Verification items for the finished model (mm, model axes). A direction names the side the tool comes from. Round coordinates to 2 decimals unless told otherwise and drop trailing zeros. Order: outer loops, then holes, each group sorted by start corner. A loop starts at its lowest first (then second) coordinate and runs counter-clockwise, first axis right, second up. Notation, with made-up numbers: M -19,26.5 L -5,26.5 A20 ccw -5,60.5 Z; hole C -21.5,3.5 d7. An arc over 180 degrees is marked long. Answer as a JSON object with one key per item and string values. Group by question number.
```python
from build123d import *

# Parameters (mm, degrees)
SKETCH_1_W          = 110
SKETCH_1_H          = 20
SKETCH_1_R          = 1.7
EXTRUDE_1_DEPTH     = 4.5
SKETCH_2_W          = 20
SKETCH_2_H          = 8
EXTRUDE_2_DEPTH     = 45
SKETCH_4_W          = 10
SKETCH_4_H          = 10
EXTRUDE_3_DEPTH     = 4.5
SKETCH_5_R          = 1.9
SKETCH_5_R_2        = 1.7
CUT_EXTRUDE_1_DEPTH = 75.885745444
CUT_EXTRUDE_2_DEPTH = 1.3
CUT_EXTRUDE_3_DEPTH = 2.6
SKETCH_7_R          = 1.7
CUT_EXTRUDE_5_DEPTH = 78.673192742
CUT_EXTRUDE_6_DEPTH = 1.3
SKETCH_9_W          = 80
SKETCH_9_H          = 3
EXTRUDE_4_DEPTH     = 50
SKETCH_11_W         = 17.2
SKETCH_11_H         = 50
SKETCH_11_W_2       = 9.3
SKETCH_11_R         = 2.5
SKETCH_11_R_2       = 1.7
CUT_EXTRUDE_7_DEPTH = 90.304255218
RIB_4_REACH         = 124.026
SKETCH_12_WALL_W    = 285.10321006
SKETCH_12_WALL_H    = 2
FILLET_1_R          = 2
FILLET_2_R          = 1.5
FILLET_3_R          = 2


with BuildPart() as part:
    # 草图1 → 凸台-拉伸1 (new body)
    with BuildSketch(Plane.XY):
        with Locations((0, 10)):
            Rectangle(SKETCH_1_W, SKETCH_1_H)
        with Locations((-45, 14)):
            Circle(SKETCH_1_R, mode=Mode.SUBTRACT)
        with Locations((-30, 14)):
            Circle(SKETCH_1_R, mode=Mode.SUBTRACT)
        with Locations((-15, 14)):
            Circle(SKETCH_1_R, mode=Mode.SUBTRACT)
        with Locations((15, 14)):
            Circle(SKETCH_1_R, mode=Mode.SUBTRACT)
        with Locations((30, 14)):
            Circle(SKETCH_1_R, mode=Mode.SUBTRACT)
        with Locations((45, 14)):
            Circle(SKETCH_1_R, mode=Mode.SUBTRACT)
    extrude(amount=EXTRUDE_1_DEPTH)

    # 草图2 → 凸台-拉伸2 (add)
    with BuildSketch(Plane.XY.offset(4.5)):
        with Locations((-45, 4)):
            Rectangle(SKETCH_2_W, SKETCH_2_H)
        with Locations((45, 4)):
            Rectangle(SKETCH_2_W, SKETCH_2_H)
    extrude(amount=EXTRUDE_2_DEPTH)

    # 草图4 → 凸台-拉伸3 (add)
    with BuildSketch(Plane.XY.offset(4.5)):
        with Locations((-19.238259457, 18.6193749)):
            Rectangle(SKETCH_4_W, SKETCH_4_H)
        with Locations((31.561740543, 18.6193749)):
            Rectangle(SKETCH_4_W, SKETCH_4_H)
    extrude(amount=-EXTRUDE_3_DEPTH)

    # 草图5 → 切除-拉伸1 (cut, through all)
    with BuildSketch(Plane.XY.offset(4.5)):
        with Locations((-19.238259457, 18.6193749)):
            Circle(SKETCH_5_R)
        with Locations((31.561740543, 18.6193749)):
            Circle(SKETCH_5_R)
        with Locations((-15, 14)):
            Circle(SKETCH_5_R_2)
        with Locations((30, 14)):
            Circle(SKETCH_5_R_2)
    extrude(amount=-CUT_EXTRUDE_1_DEPTH, mode=Mode.SUBTRACT)

    # 草图3 → 切除-拉伸2 (cut)
    with BuildSketch(Plane.XY.offset(4.5)):
        Polygon((-45, 17.22), (-47.7886018, 15.61), (-47.7886018, 12.39), (-45, 10.78), (-42.2113982, 12.39), (-42.2113982, 15.61), align=None)
        Polygon((-30, 17.22), (-32.7886018, 15.61), (-32.7886018, 12.39), (-30, 10.78), (-27.2113982, 12.39), (-27.2113982, 15.61), align=None)
        Polygon((-15, 17.22), (-17.7886018, 15.61), (-17.7886018, 12.39), (-15, 10.78), (-12.2113982, 12.39), (-12.2113982, 15.61), align=None)
        Polygon((15, 17.22), (12.2113982, 15.61), (12.2113982, 12.39), (15, 10.78), (17.7886018, 12.39), (17.7886018, 15.61), align=None)
        Polygon((30, 17.22), (27.2113982, 15.61), (27.2113982, 12.39), (30, 10.78), (32.7886018, 12.39), (32.7886018, 15.61), align=None)
        Polygon((45, 17.22), (42.2113982, 15.61), (42.2113982, 12.39), (45, 10.78), (47.7886018, 12.39), (47.7886018, 15.61), align=None)
    extrude(amount=-CUT_EXTRUDE_2_DEPTH, mode=Mode.SUBTRACT)

    # 草图6 → 切除-拉伸3 (cut)
    with BuildSketch(Plane(origin=(0, 0, 0), x_dir=(-1, 0, 0), z_dir=(0, 0, -1))):
        Polygon((-34.861740543, 18.6193749), (-33.211740543, 15.761491068), (-29.911740543, 15.761491068), (-28.261740543, 18.6193749), (-29.911740543, 21.477258733), (-33.211740543, 21.477258733), align=None)
        Polygon((15.938259457, 18.6193749), (17.588259457, 15.761491068), (20.888259457, 15.761491068), (22.538259457, 18.6193749), (20.888259457, 21.477258733), (17.588259457, 21.477258733), align=None)
    extrude(amount=-CUT_EXTRUDE_3_DEPTH, mode=Mode.SUBTRACT)

    # 草图7 → 切除-拉伸5 (cut, through all)
    with BuildSketch(Plane.XZ):
        with Locations(Location((-51, 43.5, 0), (0, 0, 270))):
            Circle(SKETCH_7_R)
        with Locations(Location((-39, 43.5, 0), (0, 0, 270))):
            Circle(SKETCH_7_R)
        with Locations(Location((-45, 33.5, 0), (0, 0, 270))):
            Circle(SKETCH_7_R)
        with Locations(Location((51, 43.5, 0), (0, 0, 270))):
            Circle(SKETCH_7_R)
        with Locations(Location((39, 43.5, 0), (0, 0, 270))):
            Circle(SKETCH_7_R)
        with Locations(Location((45, 33.5, 0), (0, 0, 270))):
            Circle(SKETCH_7_R)
    extrude(amount=-CUT_EXTRUDE_5_DEPTH, mode=Mode.SUBTRACT)

    # 草图8 → 切除-拉伸6 (cut)
    with BuildSketch(Plane(origin=(0, 8, 0), x_dir=(1, 0, 0), z_dir=(0, 1, 0))):
        Polygon((51, -46.72), (53.7886018, -45.11), (53.7886018, -41.89), (51, -40.28), (48.2113982, -41.89), (48.2113982, -45.11), align=None)
        Polygon((39, -46.72), (41.7886018, -45.11), (41.7886018, -41.89), (39, -40.28), (36.2113982, -41.89), (36.2113982, -45.11), align=None)
        Polygon((45, -36.72), (47.7886018, -35.11), (47.7886018, -31.89), (45, -30.28), (42.2113982, -31.89), (42.2113982, -35.11), align=None)
        Polygon((-39, -46.72), (-36.2113982, -45.11), (-36.2113982, -41.89), (-39, -40.28), (-41.7886018, -41.89), (-41.7886018, -45.11), align=None)
        Polygon((-51, -46.72), (-48.2113982, -45.11), (-48.2113982, -41.89), (-51, -40.28), (-53.7886018, -41.89), (-53.7886018, -45.11), align=None)
        Polygon((-45, -36.72), (-42.2113982, -35.11), (-42.2113982, -31.89), (-45, -30.28), (-47.7886018, -31.89), (-47.7886018, -35.11), align=None)
    extrude(amount=-CUT_EXTRUDE_6_DEPTH, mode=Mode.SUBTRACT)

    # 草图9 → 凸台-拉伸4 (add)
    with BuildSketch(Plane.XZ):
        with Locations((-14, 1.5)):
            Rectangle(SKETCH_9_W, SKETCH_9_H)
    extrude(amount=EXTRUDE_4_DEPTH)

    # 草图11 → 切除-拉伸7 (cut, through all)
    with BuildSketch(Plane(origin=(0, 0, 0), x_dir=(-1, 0, 0), z_dir=(0, 0, -1))):
        with Locations((-17.4, -25)):
            Rectangle(SKETCH_11_W, SKETCH_11_H)
        with Locations((49.35, -25)):
            Rectangle(SKETCH_11_W_2, SKETCH_11_H)
        with Locations((21.7, -46.25)):
            Circle(SKETCH_11_R)
        with Locations((14.7, -46.25)):
            Circle(SKETCH_11_R_2)
        with Locations((28.7, -46.25)):
            Circle(SKETCH_11_R_2)
        with Locations((21.7, -39.25)):
            Circle(SKETCH_11_R_2)
        with Locations((21.7, -32.25)):
            Circle(SKETCH_11_R_2)
        with Locations((14.7, -25.25)):
            Circle(SKETCH_11_R_2)
        with Locations((21.7, -18.25)):
            Circle(SKETCH_11_R_2)
        with Locations((28.7, -25.25)):
            Circle(SKETCH_11_R_2)
        with Locations((21.7, -25.25)):
            Circle(SKETCH_11_R)
        with Locations((4.2, -35.75)):
            Circle(SKETCH_11_R_2)
    extrude(amount=-CUT_EXTRUDE_7_DEPTH, mode=Mode.SUBTRACT)

    # 草图12 wall → 筋4 (add, up to next)
    with BuildSketch(Plane(origin=(-44.7, -15, 15.5), x_dir=(0, 0.768221279597, 0.640184399664), z_dir=(0, 0.640184399664, -0.768221279597)), mode=Mode.PRIVATE) as rib_4_sk1:
        with Locations((0, 1)):
            Rectangle(SKETCH_12_WALL_W, SKETCH_12_WALL_H)
    rib_4_tool1 = extrude(rib_4_sk1.sketch, amount=RIB_4_REACH, mode=Mode.PRIVATE) - part.part
    add(rib_4_tool1.solids().sort_by_distance((-44.7, -15, 15.5))[0])

    # 圆角1
    fillet_1_edges = [part.edges().sort_by_distance(p)[0] for p in [
        (-35, 4, 4.5),
        (-45, 8, 4.5),
        (45, 8, 4.5),
        (35, 4, 4.5),
        (8.8, 0, 1.5),
        (-44.7, 0, 14),
        (-42.7, -15, 3),
        (-42.7, 0, 15.5),
    ]]
    fillet(fillet_1_edges, radius=FILLET_1_R)

    # 圆角2
    fillet_2_edges = [part.edges().sort_by_distance(p)[0] for p in [
        (-44.7, -50, 1.5),
        (8.8, -50, 1.5),
        (-24.238259457, 20, 2.25),
        (-14.238259457, 23.6193749, 2.25),
        (-14.238259457, 20, 2.25),
        (-24.238259457, 23.6193749, 2.25),
        (-55, 20, 2.25),
        (55, 20, 2.25),
        (36.561740543, 23.6193749, 2.25),
        (36.561740543, 20, 2.25),
        (26.561740543, 20, 2.25),
        (26.561740543, 23.6193749, 2.25),
    ]]
    fillet(fillet_2_edges, radius=FILLET_2_R)

    # 圆角3
    fillet_3_edges = [part.edges().sort_by_distance(p)[0] for p in [
        (-55, 4, 49.5),
        (-35, 4, 49.5),
        (55, 4, 49.5),
        (35, 4, 49.5),
    ]]
    fillet(fillet_3_edges, radius=FILLET_3_R)


solid = part.part
```
Q1. Thickness scan on line 1 (X direction, y = 4, z = 33); line 2 (Y direction, x = -4.2, z = 1.2); line 3 (X direction, y = 4, z = 43). Record the ranges inside material, lowest first. Write a range as from..to.
Q2. Cross-section at D-D, the plane x = -0.5. Record the cut outline in (y, z).
Q3. Tool access check on faces 1 (the face through (-40, 20, 2)), 2 (the face through (45, 8, 28)), 3 (the face through (-16.775, 20.068, 1.282)), 4 (the face through (-35, 4, 27)), 5 (the face through (-46.3, 12.6, 3.2)). Record the directions out of +Z, -Z, +X, -X, +Y, -Y that give a thin tool (end or side, any length) a straight path to the whole face; none if there is none.
Q4. Cross-section at C-C, the plane z = 33.5. Record the cut outline in (x, y).
Q5. Gauge pin test, flat ends, axial feed: pin 1 Ø6 at (x, y) = (-21.7, -25.25) entering from +Z; pin 2 Ø10 at (x, z) = (44, 22) entering from +Y; pin 3 Ø1.5 at (y, z) = (-33, 2) entering from +X; pin 4 Ø3 at (x, z) = (-51, 43.5) entering from +Y. Record the tip position at first contact, or that the pin passes through.
Q6. Cross-section at B-B, the plane y = -32.25. Record the cut outline in (x, z), then the cut area to 3 significant figures.
Q7. Cross-section at A-A, the plane z = 17.5. Record the cut outline in (x, y), then the cut area to 3 significant figures.
Q8. Release check for a two-part mould opening along Z. For faces 6 (the face through (-46.3, 6.7, 34.9)), 7 (the face through (30, 20, 2.6)), 8 (the face through (-18, -50, 2)) record: released by +Z, released by -Z, zero draft, split by the parting line, or undercut.
Conclusion:
{
 "1": {"line 1": "-55..-46.62, -43.38..-35, 35..43.38, 46.62..55", "line 2": "-50..-37.45, -34.05..20", "line 3": "-55..-52.62, -49.38..-40.62, -37.38..-35, 35..37.38, 40.62..49.38, 52.62..55"},
 "2": {"outline": "M -50,0 L 20,0 L 20,4.5 L 0,4.5 L 0,3 L -50,3 Z"},
 "3": {"face 1": "+Z, -Z, -X, +Y", "face 2": "+Z, +X, -X, +Y", "face 3": "-Z", "face 4": "+Z, +Y, -Y", "face 5": "+Z"},
 "4": {"outline": "M -55,0 L -46.7,0 L -46.7,6.7 L -47.79,6.7 L -47.79,8 L -55,8 Z; M -43.3,0 L -35,0 L -35,8 L -42.21,8 L -42.21,6.7 L -43.3,6.7 Z; M 35,0 L 43.3,0 L 43.3,6.7 L 42.21,6.7 L 42.21,8 L 35,8 Z; M 46.7,0 L 55,0 L 55,8 L 47.79,8 L 47.79,6.7 L 46.7,6.7 Z"},
 "5": {"pin 1": "z = 3", "pin 2": "y = 8", "pin 3": "x = 8.8", "pin 4": "through"},
 "6": {"outline": "M -44.7,0 L -23.4,0 L -23.4,3 L -44.7,3 Z; M -20,0 L 8.8,0 L 8.8,3 L -20,3 Z", "area": "150 mm2"},
 "7": {"outline": "M -55,0 L -46.7,0 A2 cw -44.7,-2 L -44.7,-12.6 L -42.7,-12.6 L -42.7,-2 A2 cw -40.7,0 L -35,0 L -35,8 L -55,8 Z; M 35,0 L 55,0 L 55,8 L 35,8 Z", "area": "347 mm2"},
 "8": {"face 6": "undercut", "face 7": "released by -Z", "face 8": "zero draft"}
}
